Autodesk Inventor part; units mm, degrees
ref_plane "Work Plane1" through (-6.5955, 0, 23.75) normal (1, 0, 0) x (0, 1, 0)
ref_plane "YZ Plane" through (0, 0, 0) normal (1, 0, 0) x (0, 1, 0)
ref_plane "XZ Plane" through (0, 0, 0) normal (0, 1, 0) x (-1, 0, 0)
sketch "Sketch1" plane through (0, 0, 0) normal (0, 1, 0) x (-1, 0, 0)
  line L0 (-20, -20) -> (20, -20)
  line L1 (20, -20) -> (20, 20)
  line L2 (20, 20) -> (-20, 20)
  line L3 (-20, 20) -> (-20, -20)
  line L4 (-20, -20) -> (20, 20) construction
  line L5 (20, -20) -> (-20, 20) construction
  line L6 (20, 0) -> (20, 5)
  line L7 (20, 0) -> (25, 0)
  line L8 (25, 0) -> (25, 7.5)
  line L9 (25, 7.5) -> (20, 5)
  line L10 (25, 0) -> (25, -7.5)
  line L11 (20, 0) -> (20, -5)
  line L12 (20, -5) -> (25, -7.5)
  line L13 (0, 20) -> (5, 20)
  line L14 (0, 20) -> (0, 25)
  line L15 (0, 25) -> (7.5, 25)
  line L16 (7.5, 25) -> (5, 20)
  line L17 (0, 25) -> (-7.5, 25)
  line L18 (0, 20) -> (-5, 20)
  line L19 (-5, 20) -> (-7.5, 25)
  line L20 (0, -20) -> (5, -20)
  line L21 (7.5, -15) -> (5, -20)
  line L22 (0, -20) -> (-5, -20)
  line L23 (0, -20) -> (0, -15)
  line L24 (0, -15) -> (7.5, -15)
  line L25 (0, -15) -> (-7.5, -15)
  line L26 (-5, -20) -> (-7.5, -15)
  line L27 (-20, 0) -> (-20, 5)
  line L28 (-20, 0) -> (-20, -5)
  line L29 (-15, 0) -> (-15, -7.5)
  line L30 (-20, -5) -> (-15, -7.5)
  line L31 (-20, 0) -> (-15, 0)
  line L32 (-15, 7.5) -> (-20, 5)
  line L33 (-15, 0) -> (-15, 7.5)
  line L34 (24.75, 0) -> (24.75, 7.0955)
  line L35 (24.75, 7.0955) -> (20.25, 4.8455)
  line L36 (20.25, 4.8455) -> (20.25, 0)
  line L37 (24.75, 0) -> (24.75, -7.0955)
  line L38 (24.75, -7.0955) -> (20.25, -4.8455)
  line L39 (20.25, -4.8455) -> (20.25, 0)
  line L40 (0, 20.25) -> (4.8455, 20.25)
  line L41 (4.8455, 20.25) -> (7.0955, 24.75)
  line L42 (7.0955, 24.75) -> (0, 24.75)
  line L43 (0, 24.75) -> (-7.0955, 24.75)
  line L44 (-7.0955, 24.75) -> (-4.8455, 20.25)
  line L45 (-4.8455, 20.25) -> (0, 20.25)
  line L46 (24.75, 7.0955) -> (20, 4.7205)
  line L47 (24.75, -7.0955) -> (20, -4.7205)
  line L48 (7.0955, 24.75) -> (4.7205, 20)
  line L49 (-7.0955, 24.75) -> (-4.7205, 20)
  line L50 (25, 0) -> (23.75, 0)
  line L51 (23.75, 0) -> (23.75, 6.875)
  line L52 (23.75, 0) -> (23.75, -6.875)
  line L53 (0, 25) -> (0, 23.75)
  line L54 (0, 23.75) -> (6.875, 23.75)
  line L55 (0, 23.75) -> (-6.875, 23.75)
  point P0 (0, 0)
  point P1 (6.5955, 23.75)
  point P2 (-6.5955, 23.75)
  point P3 (23.75, -6.5955)
  point P4 (23.75, 6.5955)
  dimension "d0" = 40
  dimension "d1" = 40
  dimension "d2" = 5
  dimension "d3" = 5
  dimension "d4" = 7.5
  dimension "d5" = 7.5
  dimension "d6" = 5
  dimension "d9" = 40
  dimension "d16" = 40
  dimension "d21" = 0.25
  dimension "d22" = 0.25
  dimension "d23" = 0.25
  dimension "d24" = 0.25
  dimension "d29" = 1.25
  dimension "d30" = 1.25
extrude "Extrusion1" add sketch "Sketch1" along normal blind 30 contours L3 L30 L29 L33 L32 L2 L1 L0 L21 L24 L25 L26 | L1 L7 L39 L47 | L49 L45 L14 L2 | L1 L46 L36 L7 | L39 L7 L52 L38 | L14 L40 L48 L2 | L44 L55 L14 L45 | L36 L35 L51 L7 | L14 L54 L41 L40
fillet "Fillet1" radius 5 4 edges at (20, 15, 20) (20, 15, -20) (-20, 15, -20) (-20, 15, 20)
fillet "Fillet2" radius 1 4 edges at (20, 15, 5) (20, 15, -5) (5, 15, -20) (-5, 15, -20)
ref_plane "Work Plane1" through (-6.5955, 0, 23.75) normal (1, 0, 0) x (0, 1, 0)
sketch "Sketch2" plane through (-6.5955, 0, 23.75) normal (1, 0, 0) x (0, 1, 0)
  line L0 (0, -3.75) -> (30, -3.75)
  line L1 (15, -3.75) -> (15, 2)
  line L2 (30, 0) -> (25, 0)
  line L3 (0, 0) -> (30, 0)
  line L4 (0, 0) -> (5, 0)
  arc A0 (30, 0) -> (0, 0) centre (15, -55.25) ccw
  line L5 (15, 2) -> (15, 1)
  arc A1 (25, 0) -> (5, 0) centre (15, -49.5) ccw
  point P0 (0, -23.75)
  dimension "d32" = 5.75
  dimension "d33" = 5
  dimension "d34" = 5
  dimension "d35" = 1
extrude "Extrusion2" add sketch "Sketch2" along normal blind 13.191 contours A1 L3 A0 L1 | L1 A0 L2 A1
fillet "Fillet3" radius 2 2 edges at (0, 30, 23.75) (0, 0, 23.75)
sketch "Sketch3" plane through (0, 30, 0) normal (0, 1, 0) x (1, 0, 0)
  point P0 (0, 0)
pattern_circular "Circular Pattern1" count 2 over 270 about axis through (0, 30, 0) along (0, 1, 0) of "Extrusion2", "Fillet3"
properties part number "base"
Verification items for the finished model (mm, model axes). A direction names the side the tool comes from. Round coordinates to 2 decimals unless told otherwise and drop trailing zeros. Order: outer loops, then holes, each group sorted by start corner. A loop starts at its lowest first (then second) coordinate and runs counter-clockwise, first axis right, second up. Notation, with made-up numbers: (27, 48) - (60, 48) arc R6 cw to (60, 53) - close; hole circle Ø11 at (9.25, -38.75). An arc over 180 degrees is marked (long way). Use CSV: the item, a comma, the result in double quotes. Start each with the question number.
1) Section check D-D, the plane x = 8.5. Record the cut outline in (y, z), plus the area to 3 significant figures.
2) Mould release check, pull along X, two halves, no side actions. Record for faces 6 (the flat face through (-11, 15, -20)), 7 (the flat face through (-21.9, 14.79, -5.67)), 8 (the flat face through (-5.67, 14.79, 21.9)): +X half, -X half, draft (parallel to the pull), parting line (faces both ways), or undercut.
3) Section check A-A, the plane z = -0.5. Record the cut outline in (x, y), plus the area to 3 significant figures.
4) Access from +Z, -Z, +X, -X, +Y, -Y to the whole of each face (thin tool, end or side, straight path). Record for faces 1 (the flat face through (5.67, 14.79, 21.9)), 2 (the cylindrical face through (19.538, 15.21, 5.775)), 3 (the flat face through (11, 15, -20)), 4 (the cylindrical face through (19, 15, -18)), 5 (the flat face through (-6.596, 15, 25)).
5) Section check C-C, the plane y = 5.75. State how many separate pieces and enclosed holes the cut face has, plus the area to 3 significant figures.
6) Section check B-B, the plane z = -17. Record the cut outline in (x, y), plus the area to 3 significant figures.
7) Go/stop test with flat-tipped pins: P1, Ø5, axis at x = 9.5, y = 15, coming from the +Z side; P2, Ø8, axis at y = 8.5, z = 11.5, coming from the -X side; P3, Ø11.5, axis at y = 18.5, z = -12, coming from the -X side; P4, Ø10, axis at x = 3.5, y = 17, coming from the +Z side. Record where each tip stops, or that it passes through.
8) Thickness scan on L1, parallel to Z at x = -6.5, y = 7.5; L2, parallel to Z at x = -14, y = 18; L3, parallel to X at y = 16.5, z = -5. Record the ranges inside material, lowest first.
Answers:
1,outline,"(0, -20) - (30, -20) - (30, 20) - (0, 20) - close"
1,area,"1,200 mm²"
2,face 6,"draft"
2,face 7,"undercut"
2,face 8,"-X half"
3,outline,"(-24.14, 1.53) arc R2 ccw to (-22.2, 0) - (15, 0) - (15, 30) - (-22.2, 30) arc R2 ccw to (-24.14, 28.47) arc R57.25 ccw to start; hole (-23.75, 5) - (-23.75, 25) arc R50.5 ccw to start"
3,area,"1,190 mm²"
4,face 1,"+X, +Y, -Y"
4,face 2,"+Y, -Y"
4,face 3,"-Z, +X, -X, +Y, -Y"
4,face 4,"-Z, +X, +Y, -Y"
4,face 5,"+Z, -X, +Y, -Y"
5,separate pieces,"3"
5,enclosed holes,"0"
5,area,"1,570 mm²"
6,outline,"(-19.58, 0) - (-6.5, 0) - (-6.5, 30) - (-19.58, 30) - close; (6.5, 0) - (19.58, 0) - (19.58, 30) - (6.5, 30) - close"
6,area,"785 mm²"
7,P1,"stops at z = 20"
7,P2,"stops at x = -20"
7,P3,"stops at x = -25.73"
7,P4,"stops at z = 25.75"
8,L1,"z = -19.99 to -17, -15 to 20, 23.56 to 23.75, 24.19 to 25.26"
8,L2,"z = -20 to 20"
8,L3,"x = -25.73 to -24.73, -23.75 to -20.56, -20 to 15"
